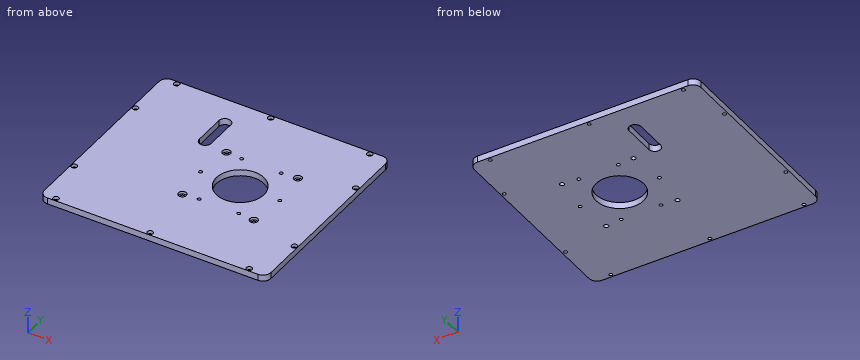
```python
from build123d import *

# Parameters (mm, degrees)
TAPA_1_4IN_START                               = 63.5
TAPA_1_4IN_DEPTH                               = 6.35
PASO_M1_ROSCA_ARO_SEPARADORES_Y_TORNILLO_START = 63.5
CROQUIS2_R                                     = 24
CROQUIS2_R_2                                   = 2.25
CROQUIS2_R_3                                   = 1.25
CROQUIS2_R_4                                   = 1.7
PASO_M1_ROSCA_ARO_SEPARADORES_Y_TORNILLO_DEPTH = 6.35
REFRENTADO_M4_CABEZA_BAJA_START                = 67.05
CROQUIS3_R                                     = 4
REFRENTADO_M4_CABEZA_BAJA_DEPTH                = 2.8
REFRENTADO_M3_START                            = 66.65
CROQUIS4_R                                     = 2.9
REFRENTADO_M3_DEPTH                            = 3.2
RANURA_CABLES_POTENCIA_CAN_START               = 63.5
RANURA_CABLES_POTENCIA_CAN_DEPTH               = 6.35
PASO_M3_ARO_TUERCA_START                       = 63.5
CROQUIS6_R                                     = 1.7
PASO_M3_ARO_TUERCA_DEPTH                       = 6.35


with BuildPart() as part:
    # Croquis1 → Tapa_1-4in (new body)
    with BuildSketch(Plane.XY.offset(TAPA_1_4IN_START)):
        with BuildLine():
            Line((-131.7, -101.6), (80.9, -101.6))
            ThreePointArc((80.9, -101.6), (86.556854249, -99.256854249), (88.9, -93.6))
            Line((88.9, -93.6), (88.9, 93.6))
            ThreePointArc((88.9, 93.6), (86.556854249, 99.256854249), (80.9, 101.6))
            Line((80.9, 101.6), (-131.7, 101.6))
            ThreePointArc((-131.7, 101.6), (-137.356854249, 99.256854249), (-139.7, 93.6))
            Line((-139.7, 93.6), (-139.7, -93.6))
            ThreePointArc((-139.7, -93.6), (-137.356854249, -99.256854249), (-131.7, -101.6))
        make_face()
    extrude(amount=TAPA_1_4IN_DEPTH)

    # Croquis2 → Paso_M1_rosca_aro_separadores_y_tornillos (cut)
    with BuildSketch(Plane.XY.offset(PASO_M1_ROSCA_ARO_SEPARADORES_Y_TORNILLO_START)):
        Circle(CROQUIS2_R)
        with Locations((-36, -36)):
            Circle(CROQUIS2_R_2)
        with Locations((-36, 36)):
            Circle(CROQUIS2_R_2)
        with Locations((36, -36)):
            Circle(CROQUIS2_R_2)
        with Locations((36, 36)):
            Circle(CROQUIS2_R_2)
        with Locations((40, 0)):
            Circle(CROQUIS2_R_3)
        with Locations((20, 34.641016151)):
            Circle(CROQUIS2_R_3)
        with Locations((-20, 34.641016151)):
            Circle(CROQUIS2_R_3)
        with Locations((-40, 0)):
            Circle(CROQUIS2_R_3)
        with Locations((-20, -34.641016151)):
            Circle(CROQUIS2_R_3)
        with Locations((20, -34.641016151)):
            Circle(CROQUIS2_R_3)
        with Locations((-125, 98.425)):
            Circle(CROQUIS2_R_4)
        with Locations((-125, -98.425)):
            Circle(CROQUIS2_R_4)
        with Locations((-30, 98.425)):
            Circle(CROQUIS2_R_4)
        with Locations((-30, -98.425)):
            Circle(CROQUIS2_R_4)
        with Locations((70, 98.425)):
            Circle(CROQUIS2_R_4)
        with Locations((70, -98.425)):
            Circle(CROQUIS2_R_4)
        with Locations((-136.525, -50)):
            Circle(CROQUIS2_R_4)
        with Locations((-136.525, 50)):
            Circle(CROQUIS2_R_4)
        with Locations((85.725, -50)):
            Circle(CROQUIS2_R_4)
        with Locations((85.725, 50)):
            Circle(CROQUIS2_R_4)
    extrude(amount=PASO_M1_ROSCA_ARO_SEPARADORES_Y_TORNILLO_DEPTH, mode=Mode.SUBTRACT)

    # Croquis3 → Refrentado_M4_cabeza_baja (cut)
    with BuildSketch(Plane.XY.offset(REFRENTADO_M4_CABEZA_BAJA_START)):
        with Locations(Location((-36, -36, 0), (0, 0, 180))):
            Circle(CROQUIS3_R)
        with Locations(Location((-36, 36, 0), (0, 0, 180))):
            Circle(CROQUIS3_R)
        with Locations(Location((36, -36, 0), (0, 0, 180))):
            Circle(CROQUIS3_R)
        with Locations(Location((36, 36, 0), (0, 0, 180))):
            Circle(CROQUIS3_R)
    extrude(amount=REFRENTADO_M4_CABEZA_BAJA_DEPTH, mode=Mode.SUBTRACT)

    # Croquis4 → Refrentado_M3 (cut)
    with BuildSketch(Plane.XY.offset(REFRENTADO_M3_START)):
        with Locations((-125, 98.425)):
            Circle(CROQUIS4_R)
        with Locations((-125, -98.425)):
            Circle(CROQUIS4_R)
        with Locations((-30, 98.425)):
            Circle(CROQUIS4_R)
        with Locations((-30, -98.425)):
            Circle(CROQUIS4_R)
        with Locations((70, 98.425)):
            Circle(CROQUIS4_R)
        with Locations((70, -98.425)):
            Circle(CROQUIS4_R)
        with Locations((-136.525, -50)):
            Circle(CROQUIS4_R)
        with Locations((-136.525, 50)):
            Circle(CROQUIS4_R)
        with Locations((85.725, -50)):
            Circle(CROQUIS4_R)
        with Locations((85.725, 50)):
            Circle(CROQUIS4_R)
    extrude(amount=REFRENTADO_M3_DEPTH, mode=Mode.SUBTRACT)

    # Croquis5 → Ranura_cables_potencia_CAN (cut)
    with BuildSketch(Plane.XY.offset(RANURA_CABLES_POTENCIA_CAN_START)):
        with BuildLine():
            Line((-66, 40), (-66, 72))
            ThreePointArc((-66, 72), (-60, 78), (-54, 72))
            Line((-54, 72), (-54, 40))
            ThreePointArc((-54, 40), (-60, 34), (-66, 40))
        make_face()
    extrude(amount=RANURA_CABLES_POTENCIA_CAN_DEPTH, mode=Mode.SUBTRACT)

    # Croquis6 → Paso_M3_aro_tuerca (cut)
    with BuildSketch(Plane.XY.offset(PASO_M3_ARO_TUERCA_START)):
        with Locations((40, 0)):
            Circle(CROQUIS6_R)
        with Locations((20, 34.641016151)):
            Circle(CROQUIS6_R)
        with Locations((-20, 34.641016151)):
            Circle(CROQUIS6_R)
        with Locations((-40, 0)):
            Circle(CROQUIS6_R)
        with Locations((-20, -34.641016151)):
            Circle(CROQUIS6_R)
        with Locations((20, -34.641016151)):
            Circle(CROQUIS6_R)
    extrude(amount=PASO_M3_ARO_TUERCA_DEPTH, mode=Mode.SUBTRACT)


solid = part.part
```
The model under review builds one solid part; all positions refer to its coordinate system, in mm. Coordinates: 2 decimals unless noted, no trailing zeros. Order: outer loops, then holes, each group sorted by start corner. A loop starts at its lowest first (then second) coordinate and runs counter-clockwise, first axis right, second up. Notation, with made-up numbers: (71.25, 15) -> (119.25, 15) arc R17 cw to (119.25, 28) -> close; hole circle Ø11 at (50, 32.25). An arc over 180 degrees is marked (long way). Answer in a Markdown table with one row per item. Add a question column.
Item 1: We need section B-B on y = 65.5. Write out the cut boundary in (x, z).
Item 2: To check wall thickness, follow probe 1 along Y at (x, z) = (-125, 65.8) (3 decimals); probe 2 along Y at (x, z) = (-36, 65.7); probe 3 along X at (y, z) = (53, 68.5). State the ranges of each line that lie inside material, in increasing order.
Item 3: We need section A-A on x = -61.5. Write out the cut boundary in (y, z).
Item 4: We need section C-C on z = 68.5. Give the number of separate pieces and of enclosed holes in the cut face, plus the area to 3 significant figures.
Item 5: Clearance check with a flat-ended pin moving along its axis: pin 1 (4.5 mm diameter, centred on x = -125, y = 98.425, fed in from +Z). State where the tip first meets the part, or that it passes through.
Final values:
| question | item | result |
|---|---|---|
| 1 | outline | (-139.7, 63.5) -> (-66, 63.5) -> (-66, 69.85) -> (-139.7, 69.85) -> close; (-54, 63.5) -> (88.9, 63.5) -> (88.9, 69.85) -> (-54, 69.85) -> close |
| 2 | probe 1 | y = -101.6 to -100.125, -96.725 to 96.725, 100.125 to 101.6 |
| 2 | probe 2 | y = -101.6 to -38.25, -33.75 to 33.75, 38.25 to 101.6 |
| 2 | probe 3 | x = -139.7 to -66, -54 to 88.9 |
| 3 | outline | (-101.6, 63.5) -> (34.19, 63.5) -> (34.19, 69.85) -> (-101.6, 69.85) -> close; (77.81, 63.5) -> (101.6, 63.5) -> (101.6, 69.85) -> (77.81, 69.85) -> close |
| 4 | separate pieces | 1 |
| 4 | enclosed holes | 22 |
| 4 | area | 43,600 mm2 |
| 5 | pin 1 | stops at z = 66.65 |
